```python
from build123d import *

# Parameters (mm, degrees)
EXTRUDE_1_DEPTH     = 15
EXTRUDE_2_DEPTH     = 4
SKETCH_3_W          = 15
SKETCH_3_H          = 5
EXTRUDE_3_DEPTH     = 4
EXTRUDE_4_DEPTH     = 2.5
SKETCH_5_W          = 22.090290278
SKETCH_5_H          = 0.2
CUT_EXTRUDE_1_DEPTH = 48.422190659


with BuildPart() as part:
    # 草图1 → 凸台-拉伸1 (new body)
    with BuildSketch(Plane.XY):
        with BuildLine():
            Line((539.301234579, 412.744075086), (539.301234579, 407.744075086))
            Line((539.301234579, 407.744075086), (534.301234579, 407.744075086))
            ThreePointArc((534.301234579, 407.744075086), (531.801234579, 410.244075086), (534.301234579, 412.744075086))
            Line((534.301234579, 412.744075086), (539.301234579, 412.744075086))
        make_face()
    extrude(amount=-EXTRUDE_1_DEPTH)

    # 草图2 → 凸台-拉伸2 (add)
    with BuildSketch(Plane(origin=(0, 0, -15), x_dir=(-1, 0, 0), z_dir=(0, 0, -1))):
        with BuildLine():
            Line((-539.301234579, 412.744075086), (-529.301234579, 412.744075086))
            ThreePointArc((-529.301234579, 412.744075086), (-526.801234579, 410.244075086), (-529.301234579, 407.744075086))
            Line((-529.301234579, 407.744075086), (-539.301234579, 407.744075086))
            Line((-539.301234579, 407.744075086), (-539.301234579, 412.744075086))
        make_face()
    extrude(amount=EXTRUDE_2_DEPTH)

    # 草图3 → 凸台-拉伸3 (add)
    with BuildSketch(Plane.XY):
        with Locations((531.801234579, 410.244075086)):
            Rectangle(SKETCH_3_W, SKETCH_3_H)
    extrude(amount=EXTRUDE_3_DEPTH)

    # 草图4 → 凸台-拉伸4 (add, symmetric)
    with BuildSketch(Plane(origin=(0, 410.244075086, 0), x_dir=(-1, 0, 0), z_dir=(0, -1, 0))):
        Polygon((-524.301234579, -4), (-537.858436246, -4), (-537.858436246, -22.261188512), (-542.306519396, -25.63298203), (-540.192207397, -28.422190659), (-533.467268804, -23.075095635), (-530.858436246, -9), align=None)
    extrude(amount=EXTRUDE_4_DEPTH, both=True)

    # 草图5 → 切除-拉伸1 (cut, through all)
    with BuildSketch(Plane(origin=(0, 0, -19), x_dir=(-1, 0, 0), z_dir=(0, 0, -1))):
        with Locations((-533.503634439, 412.644075086)):
            Rectangle(SKETCH_5_W, SKETCH_5_H)
        with Locations((-533.503634439, 407.844075086)):
            Rectangle(SKETCH_5_W, SKETCH_5_H)
    extrude(amount=-CUT_EXTRUDE_1_DEPTH, mode=Mode.SUBTRACT)


solid = part.part
```
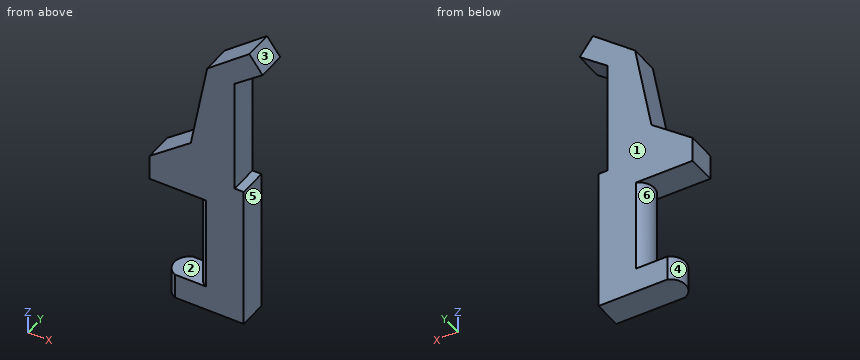
Verification items for the finished model (mm, model axes). Face numbers are marked on the shaded views. A direction names the side the tool comes from. Round coordinates to 2 decimals unless told otherwise and drop trailing zeros. Write each loop counter-clockwise with the first axis right and the second up, starting at its lowest first coordinate (ties: lowest second). Pieces come first, ordered by that corner, then holes.
1. Scan lines: L1, parallel to X at y = 412.2, z = 1; L2, parallel to Z at x = 527.5, y = 410.95; L3, parallel to Z at x = 538.75, y = 411.65. Record each from-to range of solid material in increasing order.
2. Section check B-B on y = 410.7. Enter the section's corners in (x, z).
3. Gauge pin test, flat ends, axial feed: P1, Ø1, axis at x = 538.5, y = 410.5, coming from the +Z side; P2, Ø2, axis at x = 527.5, z = -13, coming from the +Y side; P3, Ø1.5, axis at x = 528, y = 410.5, coming from the +Z side; P4, Ø0.7, axis at x = 538.5, y = 409.5, coming from the +Z side (3 decimals). Record the tip position at first contact, or that the pin passes through.
4. Section check C-C on z = -14. Enter the section's corners in (x, y).
5. Section check A-A on x = 530. Enter the section's corners in (y, z).
6. Draft check along Z on the marked faces 1, 2 and 3. Enter one of: +Z half, -Z half, draft (parallel to the pull), parting line (faces both ways), or undercut.
7. Section check D-D on x = 540.75. Enter the section's corners in (y, z).
8. Access from +Z, -Z, +X, -X, +Y, -Y to the whole of each face (thin tool, end or side, straight path). Record for the marked faces 4, 5 and 6.
Answer:
1. L1: x = 524.3 to 539.3
1. L2: z = -19 to -15, 0 to 6.44
1. L3: z = -19 to 4, 22.94 to 27.28
2. outline: (524.3, 0) - (531.84, 0) - (531.84, -15) - (526.84, -15) - (526.84, -19) - (539.3, -19) - (539.3, 4) - (537.86, 4) - (537.86, 22.26) - (542.31, 25.63) - (540.19, 28.42) - (533.47, 23.08) - (530.86, 9) - (524.3, 4) - close
3. P1: stops at z = 27.47
3. P2: passes through
3. P3: stops at z = 7.39
3. P4: stops at z = 27.355
4. outline: (533.32, 407.94) - (539.3, 407.94) - (539.3, 412.54) - (533.32, 412.54) arc R2.5 ccw to start
5. outline: (407.94, -19) - (412.54, -19) - (412.54, -15) - (407.94, -15) - close; (407.94, 0) - (412.54, 0) - (412.54, 8.35) - (407.94, 8.35) - close
6. face 1: draft
6. face 2: undercut
6. face 3: +Z half
7. outline: (407.94, 24.45) - (412.54, 24.45) - (412.54, 27.69) - (407.94, 27.69) - close
8. face 4: -Z, -X
8. face 5: -Z, +X, +Y, -Y
8. face 6: -X
